Geometry: final body of the model. Coordinates: model frame, mm. Face numbers are marked on the shaded views. A direction names the side the tool comes from. Round coordinates to 2 decimals unless told otherwise and drop trailing zeros. Loops run counter-clockwise (first coordinate to the right, second up) from the corner with the lowest first, then second, coordinate; pieces in that order, holes last. Notation, with made-up numbers: (-31.5, -27) - (-20.5, -27) arc R19 cw to (-20.5, -10) - close; hole circle Ø1 at (69, 65.5). An arc over 180 degrees is marked (long way). Answer as a JSON object with one key per item and string values. Group by question number.
Item 1: Line query: line 1 (Y direction, x = 36, z = 12.7) (3 decimals); line 2 (Z direction, x = 9.5, y = 20.5); line 3 (X direction, y = 42.5, z = 35.5). Output: solid intervals per line, ascending.
Item 2: Section D-D (x = 62). Return the cut outline in (y, z) (3 decimals).
Item 3: Section A-A (x = 49.5). Return the cut outline in (y, z) (3 decimals).
Item 4: Reachability of the marked faces 1, 2 and 3 from +Z, -Z, +X, -X, +Y, -Y: full face, straight path, thin tool, end or side. Return the list, or none.
Item 5: Draft query along Y for the marked faces 4, 5, 6 and 7. Return one class per face: released by +Y, released by -Y, zero draft, split by the parting line, or undercut.
Item 6: First-contact query: pin 1 (14 mm diameter, centred on y = 20.5, z = 41.5, fed in from +X); pin 2 (6.5 mm diameter, centred on x = 32.5, y = 41, fed in from +Z); pin 3 (7.5 mm diameter, centred on x = 35, z = 38, fed in from +Y). Flat tips, straight axial feed; report the tip coordinate or a pass-through.
Item 7: Section C-C (y = 19). Return the cut outline in (x, z), plus the area to 3 significant figures.
Item 8: Section B-B (z = 44.5). Return the cut outline in (x, y), plus the area to 3 significant figures.
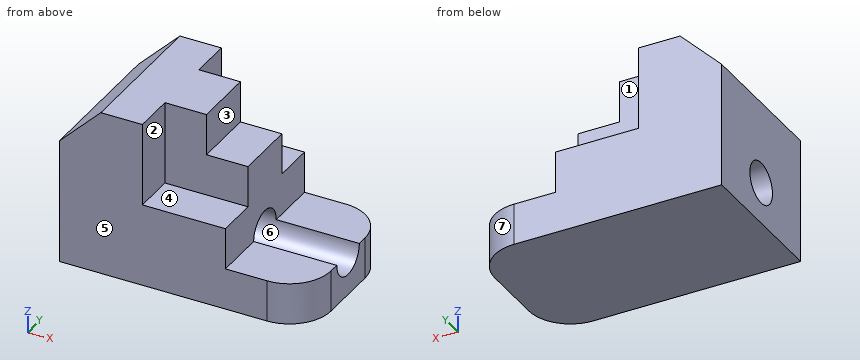
```python
from build123d import *

# Parameters (mm, degrees)
F1_DEPTH = 50.8
F3_DEPTH = 25.4
F4_DEPTH = 38.1
F2_W     = 12.7
F2_H     = 19.05
F5_DEPTH = 12.7
F7_DEPTH = 44.45
F8_R     = 6.35
F9_DEPTH = 76.2


with BuildPart() as f1:
    # F0 (on Top) → F1 (new body)
    with BuildSketch(Plane.XY):
        with BuildLine():
            Line((0, 44.45), (0, 0))
            Line((0, 0), (63.5, 0))
            ThreePointArc((63.5, 0), (72.480256, 3.719744), (76.2, 12.7))
            Line((76.2, 12.7), (76.2, 31.75))
            ThreePointArc((76.2, 31.75), (72.480256, 40.730256), (63.5, 44.45))
            Line((63.5, 44.45), (0, 44.45))
        make_face()
    extrude(amount=F1_DEPTH)

    # F2 (on face) → F3 (cut)
    with BuildSketch(Plane.XY.offset(50.8)):
        Polygon((50.8, 44.45), (25.4, 44.45), (25.4, 31.75), (38.1, 31.75), (50.8, 31.75), align=None)
        Polygon((50.8, 0), (50.8, 12.7), (38.1, 12.7), (25.4, 12.7), (25.4, 0), align=None)
    extrude(amount=-F3_DEPTH, mode=Mode.SUBTRACT)

    # F2 (on face) → F4 (cut)
    with BuildSketch(Plane.XY.offset(50.8)):
        with BuildLine():
            Line((63.5, 44.45), (50.8, 44.45))
            Line((50.8, 44.45), (50.8, 31.75))
            Line((50.8, 31.75), (50.8, 12.7))
            Line((50.8, 12.7), (50.8, 0))
            Line((50.8, 0), (63.5, 0))
            ThreePointArc((63.5, 0), (72.480256, 3.719744), (76.2, 12.7))
            Line((76.2, 12.7), (76.2, 31.75))
            ThreePointArc((76.2, 31.75), (72.480256, 40.730256), (63.5, 44.45))
        make_face()
    extrude(amount=-F4_DEPTH, mode=Mode.SUBTRACT)

    # F2 (on face) → F5 (cut)
    with BuildSketch(Plane.XY.offset(50.8)):
        with Locations((44.45, 22.225)):
            Rectangle(F2_W, F2_H)
    extrude(amount=-F5_DEPTH, mode=Mode.SUBTRACT)

    # F6 (on face) → F7 (cut, through all)
    with BuildSketch(Plane.XZ):
        Polygon((0, 50.8), (0, 38.1), (12.7, 50.8), align=None)
    extrude(amount=-F7_DEPTH, mode=Mode.SUBTRACT)

    # F8 (on face) → F9 (cut, through all)
    with BuildSketch(Plane(origin=(0, 0, 0), x_dir=(0, -1, 0), z_dir=(-1, 0, 0))):
        with Locations((-22.225, 12.7)):
            Circle(F8_R)
    extrude(amount=-F9_DEPTH, mode=Mode.SUBTRACT)


solid = f1.part
```
Values:
{
 "1": {"line 1": "y = 0 to 15.875, 28.575 to 44.45", "line 2": "z = 0 to 6.59, 18.81 to 47.6", "line 3": "x = 0 to 25.4"},
 "2": {"outline": "(0, 0) - (44.45, 0) - (44.45, 12.7) - (28.575, 12.7) arc R6.35 cw to (15.875, 12.7) - (0, 12.7) - close"},
 "3": {"outline": "(0, 0) - (44.45, 0) - (44.45, 25.4) - (31.75, 25.4) - (31.75, 38.1) - (12.7, 38.1) - (12.7, 25.4) - (0, 25.4) - close; hole circle Ø12.7 at (22.225, 12.7)"},
 "4": {"face 1": "+Z, +X, +Y", "face 2": "+Z, +X, -Y", "face 3": "+Z, +X, +Y, -Y"},
 "5": {"face 4": "zero draft", "face 5": "released by -Y", "face 6": "undercut", "face 7": "released by +Y"},
 "6": {"pin 1": "stops at x = 50.8", "pin 2": "stops at z = 25.4", "pin 3": "stops at y = 31.75"},
 "7": {"outline": "(0, 0) - (76.2, 0) - (76.2, 7.23) - (0, 7.23) - close; (0, 18.17) - (50.8, 18.17) - (50.8, 38.1) - (38.1, 38.1) - (38.1, 50.8) - (12.7, 50.8) - (0, 38.1) - close", "area": "1,970 mm^2"},
 "8": {"outline": "(6.4, 0) - (25.4, 0) - (25.4, 12.7) - (38.1, 12.7) - (38.1, 31.75) - (25.4, 31.75) - (25.4, 44.45) - (6.4, 44.45) - close", "area": "1,090 mm^2"}
}
